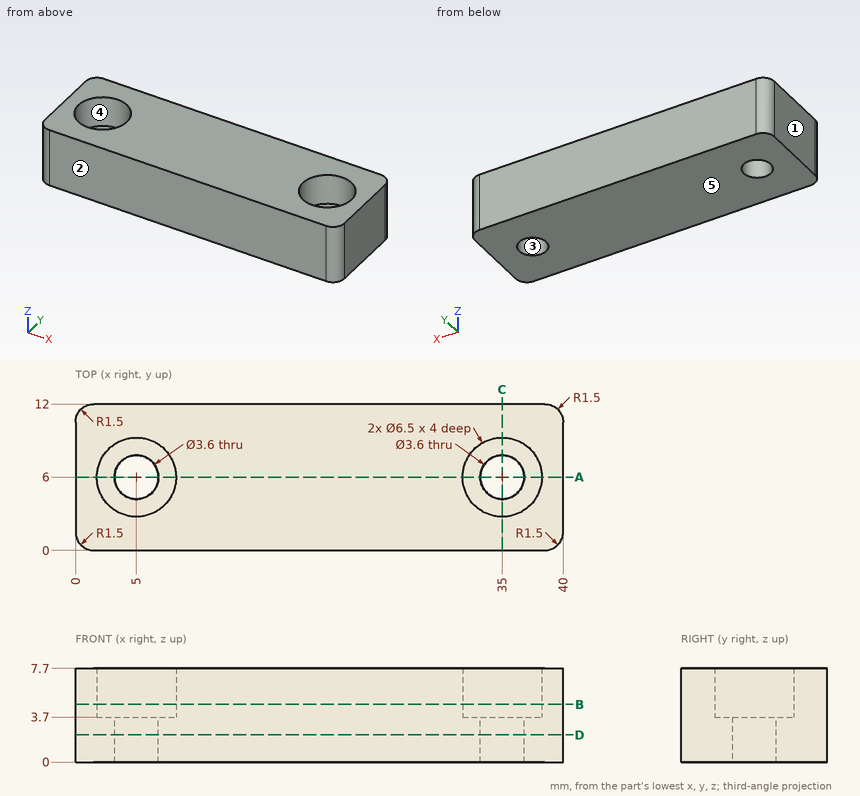
Part print with two shaded views. Sizes in mm from the minimum x, y, z corner. A direction names the side the tool comes from. Round coordinates to 2 decimals unless told otherwise and drop trailing zeros. Write each loop counter-clockwise with the first axis right and the second up, starting at its lowest first coordinate (ties: lowest second). Pieces come first, ordered by that corner, then holes. Notation, with made-up numbers: M 34.5,70.25 L 61.5,70.25 A18 cw 61.5,97.25 Z; hole C 74.5,42.25 d6. An arc over 180 degrees is marked long. Put each result on its own line as item: value. Start each with the question number.
1) Pull direction X, two halves, no side cores. Call the marked faces 1, 2 and 3: pulls with the +X half, pulls with the -X half, needs draft (parallel to the pull), parting line crosses it, or undercut.
2) Saw through at B-B, the plane z = 4.75. Write the cut outline in (x, y), and give its area (3 significant figures).
3) Drill centre lines: probe 1 along X at (y, z) = (6, 1.05); probe 2 along X at (y, z) = (6, 6.75); probe 3 along Y at (x, z) = (5, 5.85). Where is each one in solid material? Low to high. Write a range as [from, to].
4) 3-axis set-ups, long thin cutter, end or side, ignore diameter. For the marked faces 4 and 5: which of +Z, -Z, +X, -X, +Y, -Y reach the whole face in a straight line?
5) Saw through at A-A, the plane y = 6. Write the cut outline in (x, z).
6) Saw through at C-C, the plane x = 35. Write the cut outline in (y, z).
7) Saw through at D-D, the plane z = 2.25. Write the cut outline in (x, y).
8) Pin check, flat tip, straight feed: pin 1 Ø2 at (x, y) = (4.5, 7) entering from +Z. Stop position of the tip, or through.
Resolved:
1. face 1: pulls with the -X half
1. face 2: needs draft
1. face 3: undercut
2. outline: M 0,1.5 A1.5 ccw 1.5,0 L 38.5,0 A1.5 ccw 40,1.5 L 40,10.5 A1.5 ccw 38.5,12 L 1.5,12 A1.5 ccw 0,10.5 Z; hole C 5,6 d6.5; hole C 35,6 d6.5
2. area: 412 mm²
3. probe 1: [0, 3.2], [6.8, 33.2], [36.8, 40]
3. probe 2: [0, 1.75], [8.25, 31.75], [38.25, 40]
3. probe 3: [0, 2.75], [9.25, 12]
4. face 4: +Z
4. face 5: -Z, +X, -X, +Y, -Y
5. outline: M 0,0 L 3.2,0 L 3.2,3.7 L 1.75,3.7 L 1.75,7.7 L 0,7.7 Z; M 6.8,0 L 33.2,0 L 33.2,3.7 L 31.75,3.7 L 31.75,7.7 L 8.25,7.7 L 8.25,3.7 L 6.8,3.7 Z; M 36.8,0 L 40,0 L 40,7.7 L 38.25,7.7 L 38.25,3.7 L 36.8,3.7 Z
6. outline: M 0,0 L 4.2,0 L 4.2,3.7 L 2.75,3.7 L 2.75,7.7 L 0,7.7 Z; M 7.8,0 L 12,0 L 12,7.7 L 9.25,7.7 L 9.25,3.7 L 7.8,3.7 Z
7. outline: M 0,1.5 A1.5 ccw 1.5,0 L 38.5,0 A1.5 ccw 40,1.5 L 40,10.5 A1.5 ccw 38.5,12 L 1.5,12 A1.5 ccw 0,10.5 Z; hole C 5,6 d3.6; hole C 35,6 d3.6
8. pin 1: z = 3.7
